Design review of the part shown in the three views and the two pictorial views. Dimensions are in mm from the part's minimum x, y and z. A direction names the side the tool comes from. Round coordinates to 2 decimals unless told otherwise and drop trailing zeros. Order: outer loops, then holes, each group sorted by start corner. A loop starts at its lowest first (then second) coordinate and runs counter-clockwise, first axis right, second up. Notation, with made-up numbers: (41, 88) -> (89, 88) arc R25 cw to (89, 113) -> close; hole circle Ø9 at (-2.75, 88). An arc over 180 degrees is marked (long way). Put each result on its own line as item: value. Start each with the question number.
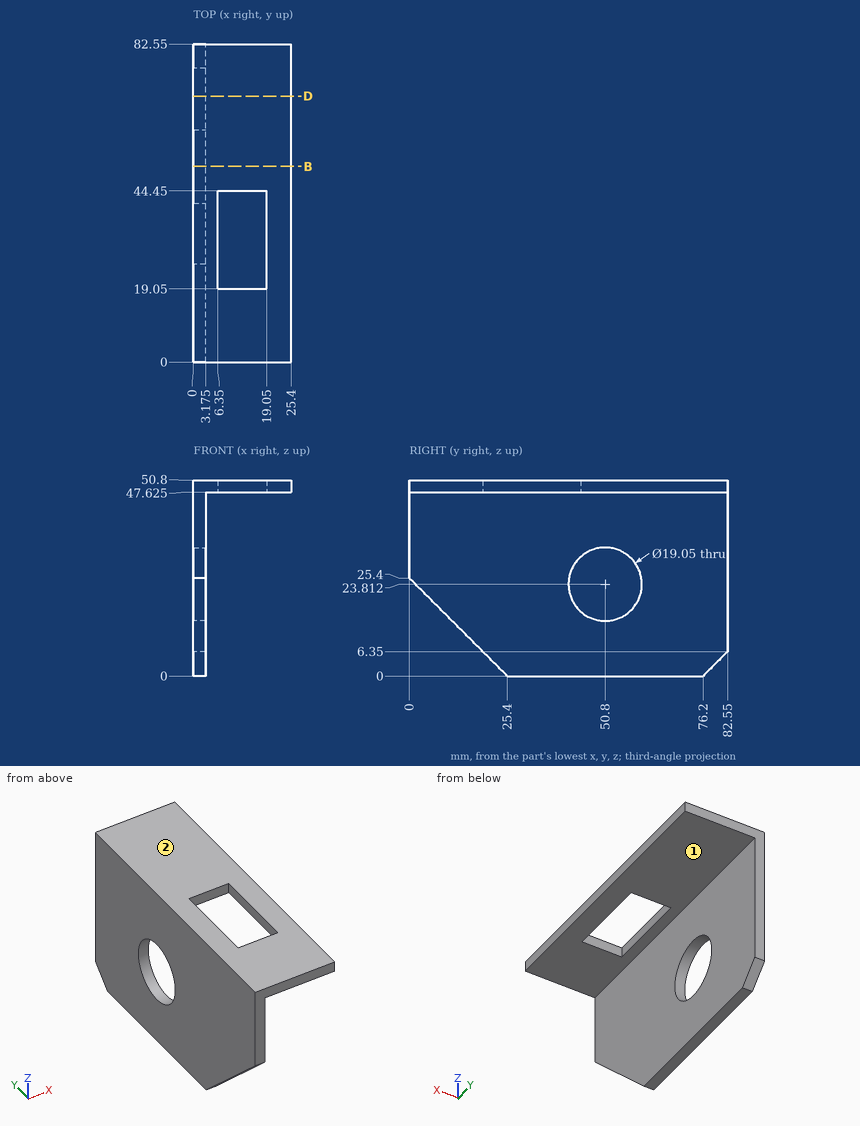
Q1. Wall thickness on probe 1 along X at (y, z) = (75, 43) (1 decimal); probe 2 along Z at (x, y) = (22.25, 48.5) (1 decimal); probe 3 along Y at (x, z) = (3, 5.5): over which ranges is each line inside the solid? List them lowest first. Write a range as [from, to].
Q2. For the marked faces 1 and 2, list the 3-axis set-ups (+Z, -Z, +X, -X, +Y, -Y) from which the entire face can be reached by the end or side of a thin tool; tool diameter is ignored.
Q3. Take a section at B-B on y = 50.8. Give the boundary of the cut face in (x, z) (1 decimal), and give its area (3 significant figures).
Q4. Clearance check with flat-ended pins moving along their axes: pin 1 Ø12 at (y, z) = (44, 24.5) entering from +X (1 decimal); pin 2 Ø11.5 at (y, z) = (50.8, 23.81) entering from -X; pin 3 Ø10 at (x, y) = (20, 13.5) entering from -Z (1 decimal). State where each tip first meets the part, or that it passes through.
Q5. Take a section at D-D on y = 69. Give the boundary of the cut face in (x, z) (1 decimal), and give its area (3 significant figures).
Calculated:
1. probe 1: x = [0, 3.2]
1. probe 2: z = [47.6, 50.8]
1. probe 3: y = [19.9, 81.7]
2. face 1: -Z, +X, +Y, -Y
2. face 2: +Z, +X, -X, +Y, -Y
3. outline: (0, 0) -> (3.2, 0) -> (3.2, 14.3) -> (0, 14.3) -> close; (0, 33.3) -> (3.2, 33.3) -> (3.2, 47.6) -> (25.4, 47.6) -> (25.4, 50.8) -> (0, 50.8) -> close
3. area: 171 mm²
4. pin 1: stops at x = 3.2
4. pin 2: passes through
4. pin 3: stops at z = 47.6
5. outline: (0, 0) -> (3.2, 0) -> (3.2, 47.6) -> (25.4, 47.6) -> (25.4, 50.8) -> (0, 50.8) -> close
5. area: 232 mm²
